```python
from build123d import *

# Parameters (mm, degrees)
F0_W     = 45.5
F0_H     = 27
F1_DEPTH = 1
F0_W_2   = 47.5
F0_H_2   = 29
F2_DEPTH = 17
F3_W     = 7
F3_H     = 8
F4_DEPTH = 17.001


with BuildPart() as f1:
    # F0 (on Top) → F1 (new body)
    with BuildSketch(Plane.XY):
        with Locations((-2.069812, 0.198113)):
            Rectangle(F0_W, F0_H)
    extrude(amount=F1_DEPTH)

    # F0 (on Top) → F2 (join)
    with BuildSketch(Plane.XY):
        with Locations((-2.069812, 0.198113)):
            Rectangle(F0_W_2, F0_H_2)
        with Locations((-2.069812, 0.198113)):
            Rectangle(F0_W, F0_H, mode=Mode.SUBTRACT)
    extrude(amount=F2_DEPTH)

    # F3 (on face) → F4 (cut, through all)
    with BuildSketch(Plane.XY):
        with Locations((-18.319812, -3.301887)):
            Rectangle(F3_W, F3_H)
    extrude(amount=F4_DEPTH, mode=Mode.SUBTRACT)


solid = f1.part
```
Design review of the part built by this model. Coordinates are the model's own, in mm. A direction names the side the tool comes from. Coordinates: 2 decimals unless noted, no trailing zeros. Order: outer loops, then holes, each group sorted by start corner. A loop starts at its lowest first (then second) coordinate and runs counter-clockwise, first axis right, second up. Notation, with made-up numbers: (-27, 51) - (28, 51) arc R28 ccw to (28, 73) - close; hole circle Ø2 at (39, 44). An arc over 180 degrees is marked (long way). Answer in a Markdown table with one row per item.
(1) Consider section A-A on z = 5.75. State the section outline as (x, y) points.
Checked values:
| item | result |
|---|---|
| outline | (-25.82, -14.3) - (21.68, -14.3) - (21.68, 14.7) - (-25.82, 14.7) - close; hole (-24.82, -13.3) - (20.68, -13.3) - (20.68, 13.7) - (-24.82, 13.7) - close |
(2) Clearance check with a flat-ended pin moving along its axis: pin 1 (8 mm diameter, centred on x = 14, y = 7, fed in from +Z). State where the tip first meets the part, or that it passes through.
Checked values:
| item | result |
|---|---|
| pin 1 | z = 1 |
(3) Consider section D-D on y = 4.25. State the section outline as (x, z) points, plus the area to 3 significant figures.
Checked values:
| item | result |
|---|---|
| outline | (-25.82, 0) - (21.68, 0) - (21.68, 17) - (20.68, 17) - (20.68, 1) - (-24.82, 1) - (-24.82, 17) - (-25.82, 17) - close |
| area | 79.5 mm^2 |
(4) Consider section C-C on x = -4. State the section outline as (y, z) points.
Checked values:
| item | result |
|---|---|
| outline | (-14.3, 0) - (14.7, 0) - (14.7, 17) - (13.7, 17) - (13.7, 1) - (-13.3, 1) - (-13.3, 17) - (-14.3, 17) - close |
(5) For faces 4 (the flat face through (-4, -14, 17)), 5 (the flat face through (-2, -13.302, 9)), 6 (the flat face through (-14.82, -3.4, 0.5)), list the 3-axis set-ups (+Z, -Z, +X, -X, +Y, -Y) from which the entire face can be reached by the end or side of a thin tool; tool diameter is ignored.
Checked values:
| item | result |
|---|---|
| face 4 | +Z, +X, -X, +Y, -Y |
| face 5 | +Z |
| face 6 | +Z, -Z |
(6) Consider section B-B on y = -2.5. State the section outline as (x, z) points, plus the area to 3 significant figures.
Checked values:
| item | result |
|---|---|
| outline | (-25.82, 0) - (-21.82, 0) - (-21.82, 1) - (-24.82, 1) - (-24.82, 17) - (-25.82, 17) - close; (-14.82, 0) - (21.68, 0) - (21.68, 17) - (20.68, 17) - (20.68, 1) - (-14.82, 1) - close |
| area | 72.5 mm^2 |
(7) Wall thickness on line 1 along Y through (x, z) = (-4.5, 15.75); line 2 along X through (y, z) = (9.75, 9.25); line 3 along Z through (x, y) = (7, 9.25): over which ranges is each line inside the solid? List them lowest first. Write a range as from..to.
Checked values:
| item | result |
|---|---|
| line 1 | -14.3..-13.3, 13.7..14.7 |
| line 2 | -25.82..-24.82, 20.68..21.68 |
| line 3 | 0..1 |
(8) The part is to be moulded in two halves that separate along Y. For faces 1 (the flat face through (-2, 0, 0)), 2 (the flat face through (-2, -14.302, 8)), 3 (the flat face through (-18.4, -7.302, 0.5)), say which applies: released by +Y, released by -Y, zero draft, split by the parting line, or undercut.
Checked values:
| item | result |
|---|---|
| face 1 | zero draft |
| face 2 | released by -Y |
| face 3 | undercut |
